from build123d import *

# Parameters (mm, degrees)
SKETCH1_W           = 95
SKETCH1_H           = 95
BOSS_EXTRUDE1_DEPTH = 25
SKETCH2_R           = 7.75
CUT_EXTRUDE2_DEPTH  = 100
SKETCH3_R           = 17
CUT_EXTRUDE3_DEPTH  = 22
CUT_EXTRUDE4_START  = -22
SKETCH4_R           = 17
CUT_EXTRUDE4_DEPTH  = 22
SKETCH5_W           = 6.246993927
SKETCH5_H           = 25
CUT_EXTRUDE5_DEPTH  = 22
SKETCH6_W           = 7.178723585
SKETCH6_H           = 25
CUT_EXTRUDE6_DEPTH  = 22
SKETCH8_W           = 99.503929421
SKETCH8_H           = 3.5
CUT_EXTRUDE7_DEPTH  = 100
SKETCH9_W           = 8.3
SKETCH9_H           = 15.5
CUT_EXTRUDE11_DEPTH = 100
SKETCH13_W          = 87
SKETCH13_H          = 15.5
CUT_EXTRUDE12_DEPTH = 2
SKETCH14_W          = 25.5
SKETCH14_H          = 47
CUT_EXTRUDE14_DEPTH = 18.5
SKETCH16_W          = 24.75
SKETCH16_H          = 47
CUT_EXTRUDE15_DEPTH = 5
SKETCH17_W          = 20.919567191
SKETCH17_H          = 47
CUT_EXTRUDE16_DEPTH = 5
CUT_EXTRUDE17_DEPTH = 100
FILLET6_R           = 1.5
FILLET7_R           = 1.5
FILLET8_R           = 1.5
FILLET9_R           = 1.5


with BuildPart() as part:
    # Sketch1 → Boss-Extrude1 (new body)
    with BuildSketch(Plane(origin=(0, 0, 0), x_dir=(1, 0, 0), z_dir=(0, 1, 0))):
        with Locations((3.271948822, -17.506298191)):
            Rectangle(SKETCH1_W, SKETCH1_H)
    extrude(amount=BOSS_EXTRUDE1_DEPTH)

    # Sketch2 → Cut-Extrude2 (cut)
    with BuildSketch(Plane.XY.offset(65.006298191)):
        with Locations((-29.228051178, 10.75)):
            Circle(SKETCH2_R)
        with Locations((15.771948822, 10.75)):
            Circle(SKETCH2_R)
    extrude(amount=-CUT_EXTRUDE2_DEPTH, mode=Mode.SUBTRACT)

    # Sketch3 → Cut-Extrude3 (cut)
    with BuildSketch(Plane.XY.offset(65.006298191)):
        with Locations((-29.228051178, 10.75)):
            Circle(SKETCH3_R)
        with Locations((15.771948822, 10.75)):
            Circle(SKETCH3_R)
    extrude(amount=-CUT_EXTRUDE3_DEPTH, mode=Mode.SUBTRACT)

    # Sketch4 → Cut-Extrude4 (cut)
    with BuildSketch(Plane(origin=(0, 0, -29.993701809), x_dir=(-1, 0, 0), z_dir=(0, 0, -1)).offset(CUT_EXTRUDE4_START)):
        with Locations((-15.771948822, 10.75)):
            Circle(SKETCH4_R)
        with Locations((29.228051178, 10.75)):
            Circle(SKETCH4_R)
    extrude(amount=CUT_EXTRUDE4_DEPTH, mode=Mode.SUBTRACT)

    # Sketch5 → Cut-Extrude5 (cut)
    with BuildSketch(Plane.XY.offset(65.006298191)):
        with Locations((-41.104554214, 12.5)):
            Rectangle(SKETCH5_W, SKETCH5_H)
    extrude(amount=-CUT_EXTRUDE5_DEPTH, mode=Mode.SUBTRACT)

    # Sketch6 → Cut-Extrude6 (cut)
    with BuildSketch(Plane(origin=(0, 0, -29.993701809), x_dir=(-1, 0, 0), z_dir=(0, 0, -1))):
        with Locations((40.638689386, 12.5)):
            Rectangle(SKETCH6_W, SKETCH6_H)
    extrude(amount=-CUT_EXTRUDE6_DEPTH, mode=Mode.SUBTRACT)

    # Sketch8 → Cut-Extrude7 (cut)
    with BuildSketch(Plane(origin=(0, 0, -29.993701809), x_dir=(-1, 0, 0), z_dir=(0, 0, -1))):
        with Locations((-1.019984112, 23.25)):
            Rectangle(SKETCH8_W, SKETCH8_H)
    extrude(amount=-CUT_EXTRUDE7_DEPTH, mode=Mode.SUBTRACT)

    # Sketch9 → Cut-Extrude11 (cut)
    with BuildSketch(Plane.XY.offset(65.006298191)):
        with Locations((-7.828051178, 10.75)):
            Rectangle(SKETCH9_W, SKETCH9_H)
    extrude(amount=-CUT_EXTRUDE11_DEPTH, mode=Mode.SUBTRACT)

    # Sketch13 → Cut-Extrude12 (cut)
    with BuildSketch(Plane.ZY.offset(3.678051178)):
        with Locations((17.506298191, 10.75)):
            Rectangle(SKETCH13_W, SKETCH13_H)
    extrude(amount=-CUT_EXTRUDE12_DEPTH, mode=Mode.SUBTRACT)

    # Sketch14 → Cut-Extrude14 (cut)
    with BuildSketch(Plane(origin=(0, 21.5, 0), x_dir=(1, 0, 0), z_dir=(0, 1, 0))):
        with Locations((-6.728051178, -17.506298191)):
            Rectangle(SKETCH14_W, SKETCH14_H)
    extrude(amount=-CUT_EXTRUDE14_DEPTH, mode=Mode.SUBTRACT)

    # Sketch16 → Cut-Extrude15 (cut)
    with BuildSketch(Plane(origin=(0, 21.5, 0), x_dir=(1, 0, 0), z_dir=(0, 1, 0))):
        with Locations((-29.853051178, -17.506298191)):
            Rectangle(SKETCH16_W, SKETCH16_H)
    extrude(amount=-CUT_EXTRUDE15_DEPTH, mode=Mode.SUBTRACT)

    # Sketch17 → Cut-Extrude16 (cut)
    with BuildSketch(Plane(origin=(0, 21.5, 0), x_dir=(1, 0, 0), z_dir=(0, 1, 0))):
        with Locations((16.481732418, -17.506298191)):
            Rectangle(SKETCH17_W, SKETCH17_H)
    extrude(amount=-CUT_EXTRUDE16_DEPTH, mode=Mode.SUBTRACT)

    # Sketch18 → Cut-Extrude17 (cut)
    with BuildSketch(Plane.XY.offset(65.006298191)):
        with BuildLine():
            Line((34.66639245, 12.75), (37.680851122, 12.75))
            ThreePointArc((37.680851122, 12.75), (37.300376381, 15.28065192), (36.628602437, 17.75))
            Line((36.628602437, 17.75), (33.435470555, 17.75))
            ThreePointArc((33.435470555, 17.75), (34.221100776, 15.291893017), (34.66639245, 12.75))
        make_face()
        with BuildLine():
            Line((34.66639245, 8.75), (37.680851122, 8.75))
            ThreePointArc((37.680851122, 8.75), (37.300376381, 6.21934808), (36.628602437, 3.75))
            Line((36.628602437, 3.75), (33.435470555, 3.75))
            ThreePointArc((33.435470555, 3.75), (34.221100776, 6.208106983), (34.66639245, 8.75))
        make_face()
    extrude(amount=-CUT_EXTRUDE17_DEPTH, mode=Mode.SUBTRACT)

    # Fillet6
    fillet6_edges = [part.edges().sort_by_distance(p)[0] for p in [
        (33.435470555, 17.75, 17.506298191),
        (36.628602437, 17.75, 17.506298191),
    ]]
    fillet(fillet6_edges, radius=FILLET6_R - 0.0001)  # a hair under: the kernel refuses the full size

    # Fillet7
    fillet7_edges = [part.edges().sort_by_distance(p)[0] for p in [
        (37.680851122, 12.75, 17.506298191),
        (34.66639245, 12.75, 17.506298191),
    ]]
    fillet(fillet7_edges, radius=FILLET7_R - 0.0001)  # a hair under: the kernel refuses the full size

    # Fillet8
    fillet8_edges = [part.edges().sort_by_distance(p)[0] for p in [
        (33.435470555, 3.75, 17.506298191),
        (36.628602437, 3.75, 17.506298191),
    ]]
    fillet(fillet8_edges, radius=FILLET8_R - 0.0001)  # a hair under: the kernel refuses the full size

    # Fillet9
    fillet9_edges = [part.edges().sort_by_distance(p)[0] for p in [
        (37.680851122, 8.75, 17.506298191),
        (34.66639245, 8.75, 17.506298191),
    ]]
    fillet(fillet9_edges, radius=FILLET9_R - 0.0001)  # a hair under: the kernel refuses the full size


solid = part.part
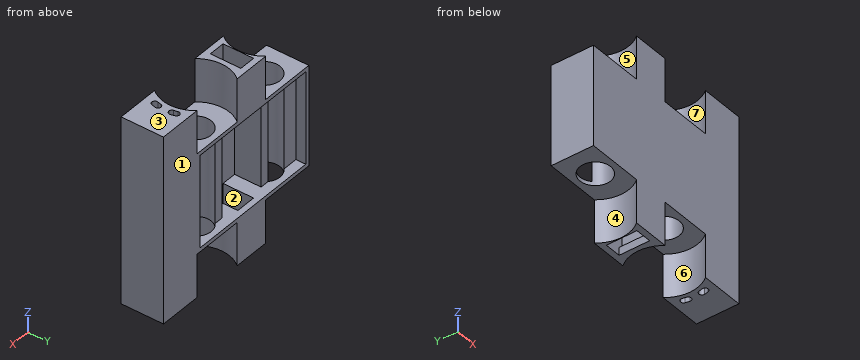
Source: CAD feature listing. Evaluate the final solid. Frame: model axes, mm. Face numbers are marked on the shaded views. A direction names the side the tool comes from. Give positions to 0.01 mm unless a question says otherwise; leave off trailing zeros. Order: outer loops, then holes, each group sorted by start corner. A loop starts at its lowest first (then second) coordinate and runs counter-clockwise, first axis right, second up. Notation, with made-up numbers: (-3.75, 0) -> (43.25, 0) arc R10 ccw to (43.25, 14) -> close; hole circle Ø1 at (21.5, -30). An arc over 180 degrees is marked (long way). Use a Markdown table: item, result.
1) Section query D-D, the plane y = 20. Return the cut outline in (x, z).
Answer list:
| item | result |
|---|---|
| outline | (-44.23, -7.99) -> (-14.96, -7.99) -> (-14.96, -29.99) -> (1.51, -29.99) -> (1.51, -7.99) -> (30.04, -7.99) -> (30.04, -29.99) -> (50.77, -29.99) -> (50.77, 65.01) -> (30.04, 65.01) -> (30.04, 43.01) -> (1.51, 43.01) -> (1.51, 65.01) -> (-14.96, 65.01) -> (-14.96, 43.01) -> (-44.23, 43.01) -> close; hole (-42.23, -5.99) -> (26.94, -5.99) -> (26.94, 41.01) -> (-42.23, 41.01) -> close |
2) Section query A-A, the plane z = 55. Count the separate pieces of the cut face and the enclosed holes in it, then the cut area to 3 significant figures.
Answer list:
| item | result |
|---|---|
| separate pieces | 2 |
| enclosed holes | 3 |
| area | 516 mm² |
3) Section query C-C, the plane x = 15.5. Return the cut outline in (y, z).
Answer list:
| item | result |
|---|---|
| outline | (0, -7.99) -> (3, -7.99) -> (3, 43.01) -> (0, 43.01) -> close; (18.5, -7.99) -> (21.5, -7.99) -> (21.5, -5.99) -> (18.5, -5.99) -> close; (18.5, 41.01) -> (21.5, 41.01) -> (21.5, 43.01) -> (18.5, 43.01) -> close |
4) Ray query, line 1 along X through (y, z) = (8, -22); line 2 along X through (y, z) = (4, -4); line 3 along X through (y, z) = (10, 7.5). Return the intervals inside material, ascending. Write a range as [from, to].
Answer list:
| item | result |
|---|---|
| line 1 | [-12.45, -11.98], [-1.68, -1], [32.55, 34.67], [37.27, 50.77] |
| line 2 | [-44.23, -33.04], [-25.42, -19.48], [6.02, 11.96], [19.58, 34.69], [36.35, 50.77] |
| line 3 | [-44.23, -36.94], [-21.51, -19.48], [6.02, 8.06], [23.49, 50.77] |
5) Contact query for flat-ended pins moving along their axis: P1, Ø5, axis at x = -22, z = 16.5, coming from the +Y side; P2, Ø6.5, axis at x = -22.5, y = 8, coming from the +Z side; P3, Ø4, axis at x = -9, y = 9, coming from the +Z side; P4, Ø12.5, axis at y = 7.5, z = 50, coming from the -X side. Output: stop coordinate, or through.
Answer list:
| item | result |
|---|---|
| P1 | y = 16.5 |
| P2 | z = 43.01 |
| P3 | through |
| P4 | x = -15.13 |
6) Mould query, pull axis Y, two halves, no side actions, for the marked faces 1, 2 and 3. Classes: +Y half, -Y half, draft (parallel to the pull), parting line (faces both ways), or undercut.
Answer list:
| item | result |
|---|---|
| face 1 | +Y half |
| face 2 | undercut |
| face 3 | draft |
7) Reachability of the marked faces 4, 5, 6 and 7 from +Z, -Z, +X, -X, +Y, -Y: full face, straight path, thin tool, end or side. Return the list, or none.
Answer list:
| item | result |
|---|---|
| face 4 | -Z, -X |
| face 5 | +Z, -X |
| face 6 | -Z |
| face 7 | +Z |
